Input: part model. Units: mm. Frame: model coordinates. Face numbers are marked on the shaded views. A direction names the side the tool comes from. Give positions to 0.01 mm unless a question says otherwise; leave off trailing zeros. Loops run counter-clockwise (first coordinate to the right, second up) from the corner with the lowest first, then second, coordinate; pieces in that order, holes last. Notation, with made-up numbers: M 59.25,34 L 117.25,34 A18 ccw 117.25,57 Z; hole C -21.5,73 d11. An arc over 180 degrees is marked long. Answer as a JSON object with one key per item and string values. Group by question number.
1) Ray query, L1, parallel to X at y = -0.3, z = -12; L2, parallel to Z at x = -8.5, y = -3.25; L3, parallel to Y at x = 11, z = -5.5. Return the intervals inside material, ascending.
2) Section query A-A on x = 15. Return loops of the section in (y, z).
3) Section query B-B on z = 12. Return loops of the section in (x, y), plus the area to 3 significant figures.
4) Draft query along Z for the marked faces 4, 5 and 6. Return one class per face: +Z half, -Z half, draft (parallel to the pull), parting line (faces both ways), or undercut.
5) Section query D-D on z = 27. Return loops of the section in (x, y).
6) First-contact query: P1, Ø3.5, axis at x = 15, z = 12, coming from the -Y side; P2, Ø1.5, axis at x = -23, y = -3, coming from the -Z side; P3, Ø9, axis at x = 0.5, z = -39.5, coming from the +Y side. Flat tips, straight axial feed; report the tip coordinate or a pass-through.
7) Access query for the marked faces 1, 2 and 3. Directions: +Z, -Z, +X, -X, +Y, -Y. A direction counts if a zero-diameter tool reaches every point of the face in a straight line with its end or side. Return the directions, or none.
8) Section query C-C on y = -6.25. Return loops of the section in (x, z).
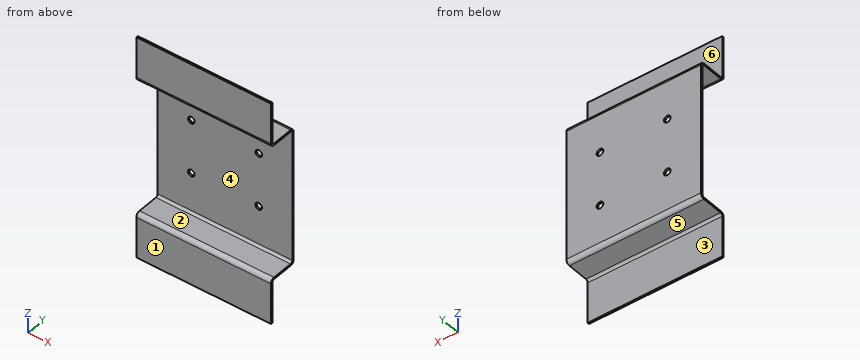
from build123d import *

# Parameters (mm, degrees)
SKETCH7_W                      = 60
SKETCH7_H                      = 60
BASE_FLANGE2_DEPTH             = 0.8
EDGE_FLANGE1_STRIP_W           = 5.2
EDGE_FLANGE1_STRIP_H           = 0.8
EDGE_FLANGE1_STRIP_CUT_DEPTH   = 60
EDGE_FLANGE1_STRIP_2_W         = 5.2
EDGE_FLANGE1_STRIP_2_H         = 0.8
EDGE_FLANGE1_STRIP_CUT_2_DEPTH = 60
EDGE_FLANGE1_DEPTH             = 60
EDGE_FLANGE1_BEND_DEPTH        = 60
EDGE_FLANGE2_STRIP_W           = 5.2
EDGE_FLANGE2_STRIP_H           = 0.8
EDGE_FLANGE2_STRIP_CUT_DEPTH   = 60
EDGE_FLANGE2_STRIP_2_W         = 5.2
EDGE_FLANGE2_STRIP_2_H         = 0.8
EDGE_FLANGE2_STRIP_CUT_2_DEPTH = 60
EDGE_FLANGE2_DEPTH             = 60
EDGE_FLANGE2_BEND_DEPTH        = 60
SKETCH22_R                     = 1.5
CUT_EXTRUDE2_DEPTH             = 60.741108125


# Sheet-metal steps are written as plain solids
with BuildPart() as part:
    # Sketch7 → Base-Flange2 (new body)
    with BuildSketch(Plane(origin=(0, 0, 0), x_dir=(1, 0, 0), z_dir=(0, 1, 0))):
        Rectangle(SKETCH7_W, SKETCH7_H)
    extrude(amount=-BASE_FLANGE2_DEPTH)

    # Edge-Flange1 strip (across the edge) → Edge-Flange1 strip cut (cut)
    with BuildSketch(Plane(origin=(-30, -0.8, -30), x_dir=(0, 0, 1), z_dir=(1, 0, 0))):
        with Locations((-1.6, -0.4)):
            Rectangle(EDGE_FLANGE1_STRIP_W, EDGE_FLANGE1_STRIP_H)
    extrude(amount=EDGE_FLANGE1_STRIP_CUT_DEPTH, mode=Mode.SUBTRACT)

    # Edge-Flange1 strip 2 (across the edge) → Edge-Flange1 strip cut 2 (cut)
    with BuildSketch(Plane(origin=(30, -0.8, 30), x_dir=(0, 0, -1), z_dir=(-1, 0, 0))):
        with Locations((-1.6, -0.4)):
            Rectangle(EDGE_FLANGE1_STRIP_2_W, EDGE_FLANGE1_STRIP_2_H)
    extrude(amount=EDGE_FLANGE1_STRIP_CUT_2_DEPTH, mode=Mode.SUBTRACT)

    # Edge-Flange1 section (across the edge) → Edge-Flange1 (add)
    with BuildSketch(Plane(origin=(-30, -0.8, -30), x_dir=(0, 0, 1), z_dir=(1, 0, 0))):
        with BuildLine():
            Line((-0.8, 1), (-0.8, 12.2))
            Line((-0.8, 12.2), (0, 12.2))
            Line((0, 12.2), (0, 1))
            ThreePointArc((0, 1), (0.292893219, 0.292893219), (1, 0))
            Line((1, 0), (1, -0.8))
            ThreePointArc((1, -0.8), (-0.272792206, -0.272792206), (-0.8, 1))
        make_face()
    extrude(amount=EDGE_FLANGE1_DEPTH)

    # Edge-Flange1 section 2 (across the edge) → Edge-Flange1 bend (add)
    with BuildSketch(Plane(origin=(30, -0.8, 30), x_dir=(0, 0, -1), z_dir=(-1, 0, 0))):
        with BuildLine():
            Line((-0.8, 1), (-0.8, 12.2))
            Line((-0.8, 12.2), (0, 12.2))
            Line((0, 12.2), (0, 1))
            ThreePointArc((0, 1), (0.292893219, 0.292893219), (1, 0))
            Line((1, 0), (1, -0.8))
            ThreePointArc((1, -0.8), (-0.272792206, -0.272792206), (-0.8, 1))
        make_face()
    extrude(amount=EDGE_FLANGE1_BEND_DEPTH)

    # Edge-Flange2 strip (across the edge) → Edge-Flange2 strip cut (cut)
    with BuildSketch(Plane(origin=(-30, -13, 30.8), x_dir=(0, 1, 0), z_dir=(1, 0, 0))):
        with Locations((-0.8, -0.4)):
            Rectangle(EDGE_FLANGE2_STRIP_W, EDGE_FLANGE2_STRIP_H)
    extrude(amount=EDGE_FLANGE2_STRIP_CUT_DEPTH, mode=Mode.SUBTRACT)

    # Edge-Flange2 strip 2 (across the edge) → Edge-Flange2 strip cut 2 (cut)
    with BuildSketch(Plane(origin=(30, -13, -30.8), x_dir=(0, 1, 0), z_dir=(-1, 0, 0))):
        with Locations((-0.8, -0.4)):
            Rectangle(EDGE_FLANGE2_STRIP_2_W, EDGE_FLANGE2_STRIP_2_H)
    extrude(amount=EDGE_FLANGE2_STRIP_CUT_2_DEPTH, mode=Mode.SUBTRACT)

    # Edge-Flange2 section (across the edge) → Edge-Flange2 (add)
    with BuildSketch(Plane(origin=(-30, -13, 30.8), x_dir=(0, 1, 0), z_dir=(1, 0, 0))):
        with BuildLine():
            Line((0, 1), (0, 19.2))
            Line((0, 19.2), (0.8, 19.2))
            Line((0.8, 19.2), (0.8, 1))
            ThreePointArc((0.8, 1), (1.092893219, 0.292893219), (1.8, 0))
            Line((1.8, 0), (1.8, -0.8))
            ThreePointArc((1.8, -0.8), (0.527207794, -0.272792206), (0, 1))
        make_face()
    extrude(amount=EDGE_FLANGE2_DEPTH)

    # Edge-Flange2 section 2 (across the edge) → Edge-Flange2 bend (add)
    with BuildSketch(Plane(origin=(30, -13, -30.8), x_dir=(0, 1, 0), z_dir=(-1, 0, 0))):
        with BuildLine():
            Line((0, 1), (0, 19.2))
            Line((0, 19.2), (0.8, 19.2))
            Line((0.8, 19.2), (0.8, 1))
            ThreePointArc((0.8, 1), (1.092893219, 0.292893219), (1.8, 0))
            Line((1.8, 0), (1.8, -0.8))
            ThreePointArc((1.8, -0.8), (0.527207794, -0.272792206), (0, 1))
        make_face()
    extrude(amount=EDGE_FLANGE2_BEND_DEPTH)

    # Sketch22 → Cut-Extrude2 (cut, through all)
    with BuildSketch(Plane(origin=(0, 0, 0), x_dir=(1, 0, 0), z_dir=(0, 1, 0))):
        with Locations(Location((-15, 12, 0), (0, 0, 270))):
            Circle(SKETCH22_R)
        with Locations(Location((15, 12, 0), (0, 0, 270))):
            Circle(SKETCH22_R)
        with Locations(Location((15, -12, 0), (0, 0, 270))):
            Circle(SKETCH22_R)
        with Locations(Location((-15, -12, 0), (0, 0, 270))):
            Circle(SKETCH22_R)
    extrude(amount=-CUT_EXTRUDE2_DEPTH, mode=Mode.SUBTRACT)


solid = part.part
Output:
{
 "1": {"L1": "x = -30 to -16.5, -13.5 to 13.5, 16.5 to 30", "L2": "z = -30.8 to -30, 30 to 30.8", "L3": "y = -0.8 to 0"},
 "2": {"outline": "M -13,-50 L -12.2,-50 L -12.2,-31.8 A1 cw -11.2,-30.8 L -1.8,-30.8 A1.8 ccw 0,-29 L 0,-13.5 L -0.8,-13.5 L -0.8,-29 A1 cw -1.8,-30 L -11.2,-30 A1.8 ccw -13,-31.8 Z; M -13,31.8 A1.8 ccw -11.2,30 L -1.8,30 A1 cw -0.8,29 L -0.8,13.5 L 0,13.5 L 0,29 A1.8 ccw -1.8,30.8 L -11.2,30.8 A1 cw -12.2,31.8 L -12.2,50 L -13,50 Z; M -0.8,-10.5 L 0,-10.5 L 0,10.5 L -0.8,10.5 Z"},
 "3": {"outline": "M -30,-0.8 L -16.5,-0.8 L -16.5,0 L -30,0 Z; M -13.5,-0.8 L 13.5,-0.8 L 13.5,0 L -13.5,0 Z; M 16.5,-0.8 L 30,-0.8 L 30,0 L 16.5,0 Z", "area": "43.2 mm^2"},
 "4": {"face 4": "undercut", "face 5": "-Z half", "face 6": "draft"},
 "5": {"outline": "M -30,-0.8 L 30,-0.8 L 30,0 L -30,0 Z"},
 "6": {"P1": "stops at y = -0.8", "P2": "stops at z = -30.8", "P3": "stops at y = -12.2"},
 "7": {"face 1": "+Z, -Z, +X, -X, -Y", "face 2": "+X, -X, -Y", "face 3": "-Z, +X, -X, +Y"},
 "8": {"outline": "M -30,-30.8 L 30,-30.8 L 30,-30 L -30,-30 Z; M -30,30 L 30,30 L 30,30.8 L -30,30.8 Z"}
}
